Work out the finished part from the listing and answer in its coordinate system (mm). A direction names the side the tool comes from. Round coordinates to 2 decimals unless told otherwise and drop trailing zeros. Order: outer loops, then holes, each group sorted by start corner. A loop starts at its lowest first (then second) coordinate and runs counter-clockwise, first axis right, second up. Notation, with made-up numbers: (-22.75, -4.75) - (34.25, -4.75) arc R20 cw to (34.25, 25.25) - close; hole circle Ø2 at (49, 34.25). An arc over 180 degrees is marked (long way). Put each result on its own line as item: value.
```python
from build123d import *

# Parameters (mm, degrees)
SKETCH_1_W      = 118
SKETCH_1_H      = 60.5
EXTRUDE_1_DEPTH = 13
FILLET_1_R      = 2
FILLET_2_R      = 2


with BuildPart() as part:
    # 草图1 → 凸台-拉伸1 (new body)
    with BuildSketch(Plane(origin=(0, 0, 0), x_dir=(1, 0, 0), z_dir=(0, 1, 0))):
        Polygon((-59, 0), (-59, 30.25), (-74, 30.25), align=None)
        Rectangle(SKETCH_1_W, SKETCH_1_H)
    extrude(amount=EXTRUDE_1_DEPTH)

    # 圆角1
    fillet_1_edges = [part.edges().sort_by_distance(p)[0] for p in [
        (-66.5, 13, -15.125),
        (-59, 13, 15.125),
        (0, 13, 30.25),
        (59, 13, 0),
        (-7.5, 13, -30.25),
    ]]
    fillet(fillet_1_edges, radius=FILLET_1_R)

    # 圆角2
    fillet_2_edges = [part.edges().sort_by_distance(p)[0] for p in [
        (59, 0, 0),
        (0, 0, 30.25),
        (-59, 0, 15.125),
        (-66.5, 0, -15.125),
        (-7.5, 0, -30.25),
    ]]
    fillet(fillet_2_edges, radius=FILLET_2_R)


solid = part.part
```
1) A cutting plane is placed at A-A on z = 4.5. Write down the section's boundary in (x, y), then the cut area to 3 significant figures.
Findings below:
outline: (-59, 2) arc R2 ccw to (-57, 0) - (57, 0) arc R2 ccw to (59, 2) - (59, 11) arc R2 ccw to (57, 13) - (-57, 13) arc R2 ccw to (-59, 11) - close
area: 1,530 mm2
2) Given pin 1 Ø4.5 at (y, z) = (6.5, 8) entering from -X; pin 2 Ø5 at (y, z) = (5, -11) entering from -X, each flat-ended and moving along its own axis, determine where each tip first touches the part or whether it passes through.
Findings below:
pin 1: stops at x = -59
pin 2: stops at x = -65.69
3) For faces 1 (the flat face through (-59, 6, 15)), 2 (the flat face through (-8, 0, 0)), determine the directions among +Z, -Z, +X, -X, +Y, -Y from which every point of the face is accessible in a straight line to the end or side of a thin tool.
Findings below:
face 1: +Z, -X, +Y, -Y
face 2: +Z, -Z, +X, -X, -Y
4) A cutting plane is placed at B-B on y = 4. Write down the section's boundary in (x, z).
Findings below:
outline: (-74, -30.25) - (59, -30.25) - (59, 30.25) - (-59, 30.25) - (-59, 0) - close
5) Straight lines are drawn through the part: L1, parallel to X at y = 6.75, z = 0.5; L2, parallel to X at y = 4.5, z = -9; L3, parallel to Z at x = -47.5, y = 1.25. For each, find the intervals that lie inside material, in ascending order. Write a range as from..to.
Findings below:
L1: x = -59..59
L2: x = -63.46..59
L3: z = -30.1..30.1
